Geometry check sheet. Reference: the model listing, model coordinates, mm. Face numbers are marked on the shaded views. Coordinates: 2 decimals unless noted, no trailing zeros. Order: outer loops, then holes, each group sorted by start corner. A loop starts at its lowest first (then second) coordinate and runs counter-clockwise, first axis right, second up. Notation, with made-up numbers: (59, 78) - (118, 78) arc R13 cw to (118, 88) - close; hole circle Ø7 at (-27, 32). An arc over 180 degrees is marked (long way). Put each result on its own line as item: value.
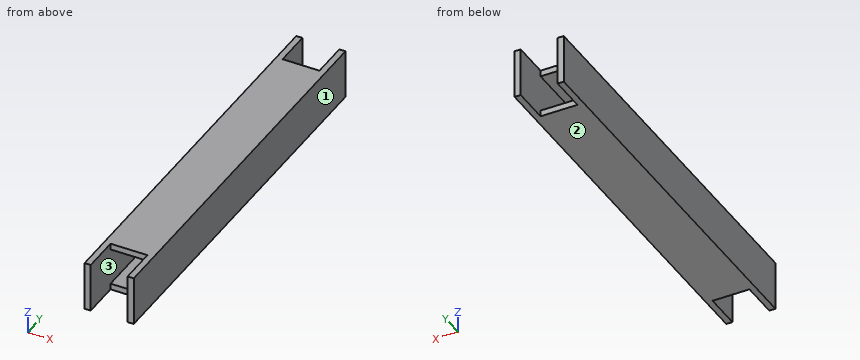
from build123d import *

# Parameters (mm, degrees)
SKETCH1_W           = 25.4
SKETCH1_H           = 25.4
SKETCH1_W_2         = 19.05
SKETCH1_H_2         = 19.05
EXTRUDE_THIN1_DEPTH = 203.2
SKETCH3_W           = 19.05
SKETCH3_H           = 19.05
CUT_EXTRUDE1_DEPTH  = 207.350575478
SKETCH4_W           = 19.05
SKETCH4_H           = 19.05
CUT_EXTRUDE2_DEPTH  = 207.350575478


with BuildPart() as part:
    # Sketch1 → Extrude-Thin1 (new body)
    with BuildSketch(Plane(origin=(0, 0, 0), x_dir=(1, 0, 0), z_dir=(0, 1, 0))):
        with Locations((12.7, 12.7)):
            Rectangle(SKETCH1_W, SKETCH1_H)
        with Locations((12.7, 12.7)):
            Rectangle(SKETCH1_W_2, SKETCH1_H_2, mode=Mode.SUBTRACT)
    extrude(amount=EXTRUDE_THIN1_DEPTH)

    # Sketch3 → Cut-Extrude1 (cut, through all)
    with BuildSketch(Plane.XY):
        with Locations((12.7, 193.675)):
            Rectangle(SKETCH3_W, SKETCH3_H)
    extrude(amount=-CUT_EXTRUDE1_DEPTH, mode=Mode.SUBTRACT)

    # Sketch4 → Cut-Extrude2 (cut, through all)
    with BuildSketch(Plane.XY):
        with Locations((12.7, 9.525)):
            Rectangle(SKETCH4_W, SKETCH4_H)
    extrude(amount=-CUT_EXTRUDE2_DEPTH, mode=Mode.SUBTRACT)


solid = part.part
Q1. Draft check along X on the marked faces 1, 2 and 3. Enter one of: pulls with the +X half, pulls with the -X half, needs draft (parallel to the pull), parting line crosses it, or undercut.
Answer block:
face 1: pulls with the +X half
face 2: needs draft
face 3: undercut
Q2. Section check C-C on y = 157.5. Record the boundary of the cut face in (x, z) (3 decimals), then the cut area to 3 significant figures.
Answer block:
outline: (0, -25.4) - (25.4, -25.4) - (25.4, 0) - (0, 0) - close; hole (3.175, -22.225) - (22.225, -22.225) - (22.225, -3.175) - (3.175, -3.175) - close
area: 282 mm^2
Q3. Section check B-B on z = -8.75. Record the boundary of the cut face in (x, y) (3 decimals).
Answer block:
outline: (0, 0) - (3.175, 0) - (3.175, 203.2) - (0, 203.2) - close; (22.225, 0) - (25.4, 0) - (25.4, 203.2) - (22.225, 203.2) - close
Q4. Thickness scan on L1, parallel to Z at x = 21, y = 28 (3 decimals); L2, parallel to X at y = 148.5, z = -10.25 (3 decimals). Record the ranges inside material, lowest first. Write a range as [from, to].
Answer block:
L1: z = [-25.4, -22.225], [-3.175, 0]
L2: x = [0, 3.175], [22.225, 25.4]
Q5. Section check A-A on y = 13. Record the boundary of the cut face in (x, z) (3 decimals), then the cut area to 3 significant figures.
Answer block:
outline: (0, -25.4) - (3.175, -25.4) - (3.175, 0) - (0, 0) - close; (22.225, -25.4) - (25.4, -25.4) - (25.4, 0) - (22.225, 0) - close
area: 161 mm^2
Q6. Depth check by flat-ended pin: pin 1 Ø1 at (x, z) = (14, -2.5) entering from -Y; pin 2 Ø2.5 at (x, z) = (13.5, -23.5) entering from +Y; pin 3 Ø2 at (x, z) = (20.5, -16.5) entering from -Y. Enter the tip coordinate at first touch or a pass-through.
Answer block:
pin 1: stops at y = 19.05
pin 2: stops at y = 184.15
pin 3: passes through
